from build123d import *

# Parameters (mm, degrees)
SKETCH_1_W          = 143
SKETCH_1_H          = 57.5
EXTRUDE_1_DEPTH     = 2
SKETCH_4_W          = 120
SKETCH_4_H          = 16
CUT_EXTRUDE_1_DEPTH = 10
FILLET_1_R          = 3
CUT_EXTRUDE_2_DEPTH = 10
SKETCH_6_W          = 32
SKETCH_6_H          = 16
EXTRUDE_2_DEPTH     = 2
CUT_EXTRUDE_3_DEPTH = 2
FILLET_2_R          = 3
FILLET_3_R          = 2
SKETCH_8_R          = 1.5
CUT_EXTRUDE_4_DEPTH = 78.089639382
SKETCH_10_R         = 1.721982437
CUT_EXTRUDE_5_DEPTH = 78.089639382
SKETCH_12_R         = 1.5
CUT_EXTRUDE_6_DEPTH = 78.089639382


with BuildPart() as part:
    # 草图1 → 凸台-拉伸1 (new body)
    with BuildSketch(Plane.XY):
        Rectangle(SKETCH_1_W, SKETCH_1_H)
    extrude(amount=EXTRUDE_1_DEPTH)

    # 草图4 → 切除-拉伸1 (cut)
    with BuildSketch(Plane(origin=(0, 0, 0), x_dir=(-1, 0, 0), z_dir=(0, 0, -1))):
        with Locations((0, -20.75)):
            Rectangle(SKETCH_4_W, SKETCH_4_H)
    extrude(amount=-CUT_EXTRUDE_1_DEPTH, mode=Mode.SUBTRACT)

    # 圆角1
    fillet_1_edges = [part.edges().sort_by_distance(p)[0] for p in [
        (-60, -28.75, 1),
        (60, -28.75, 1),
        (-71.5, 28.75, 1),
        (71.5, 28.75, 1),
        (71.5, -28.75, 1),
        (-71.5, -28.75, 1),
    ]]
    fillet(fillet_1_edges, radius=FILLET_1_R)

    # 草图5 → 切除-拉伸2 (cut)
    with BuildSketch(Plane.XY.offset(2)):
        with BuildLine():
            Line((4, 19.75), (4, 1.75))
            ThreePointArc((4, 1.75), (0, -2.25), (-4, 1.75))
            Line((-4, 1.75), (-4, 19.75))
            ThreePointArc((-4, 19.75), (0, 23.75), (4, 19.75))
        make_face()
        with BuildLine():
            Line((18, 19.75), (18, 1.75))
            ThreePointArc((18, 1.75), (14, -2.25), (10, 1.75))
            Line((10, 1.75), (10, 19.75))
            ThreePointArc((10, 19.75), (14, 23.75), (18, 19.75))
        make_face()
        with BuildLine():
            Line((32, 19.75), (32, 1.75))
            ThreePointArc((32, 1.75), (28, -2.25), (24, 1.75))
            Line((24, 1.75), (24, 19.75))
            ThreePointArc((24, 19.75), (28, 23.75), (32, 19.75))
        make_face()
        with BuildLine():
            Line((46, 19.75), (46, 1.75))
            ThreePointArc((46, 1.75), (42, -2.25), (38, 1.75))
            Line((38, 1.75), (38, 19.75))
            ThreePointArc((38, 19.75), (42, 23.75), (46, 19.75))
        make_face()
        with BuildLine():
            Line((60, 19.75), (60, 1.75))
            ThreePointArc((60, 1.75), (56, -2.25), (52, 1.75))
            Line((52, 1.75), (52, 19.75))
            ThreePointArc((52, 19.75), (56, 23.75), (60, 19.75))
        make_face()
        with BuildLine():
            Line((-60, 19.75), (-60, 1.75))
            ThreePointArc((-60, 1.75), (-56, -2.25), (-52, 1.75))
            Line((-52, 1.75), (-52, 19.75))
            ThreePointArc((-52, 19.75), (-56, 23.75), (-60, 19.75))
        make_face()
        with BuildLine():
            Line((-46, 19.75), (-46, 1.75))
            ThreePointArc((-46, 1.75), (-42, -2.25), (-38, 1.75))
            Line((-38, 1.75), (-38, 19.75))
            ThreePointArc((-38, 19.75), (-42, 23.75), (-46, 19.75))
        make_face()
        with BuildLine():
            Line((-32, 19.75), (-32, 1.75))
            ThreePointArc((-32, 1.75), (-28, -2.25), (-24, 1.75))
            Line((-24, 1.75), (-24, 19.75))
            ThreePointArc((-24, 19.75), (-28, 23.75), (-32, 19.75))
        make_face()
        with BuildLine():
            Line((-18, 19.75), (-18, 1.75))
            ThreePointArc((-18, 1.75), (-14, -2.25), (-10, 1.75))
            Line((-10, 1.75), (-10, 19.75))
            ThreePointArc((-10, 19.75), (-14, 23.75), (-18, 19.75))
        make_face()
    extrude(amount=-CUT_EXTRUDE_2_DEPTH, mode=Mode.SUBTRACT)

    # 草图6 → 凸台-拉伸2 (add)
    with BuildSketch(Plane(origin=(0, 0, 0), x_dir=(-1, 0, 0), z_dir=(0, 0, -1))):
        with Locations((0, -20.75)):
            Rectangle(SKETCH_6_W, SKETCH_6_H)
    extrude(amount=-EXTRUDE_2_DEPTH)

    # 草图7 → 切除-拉伸3 (cut)
    with BuildSketch(Plane(origin=(0, 0, 0), x_dir=(-1, 0, 0), z_dir=(0, 0, -1))):
        with BuildLine():
            Line((-10, -28.75), (10, -28.75))
            ThreePointArc((10, -28.75), (0, -18.75), (-10, -28.75))
        make_face()
    extrude(amount=-CUT_EXTRUDE_3_DEPTH, mode=Mode.SUBTRACT)

    # 圆角2
    fillet_2_edges = [part.edges().sort_by_distance(p)[0] for p in [
        (-60, -12.75, 1),
        (60, -12.75, 1),
        (-16, -12.75, 1),
        (-16, -28.75, 1),
        (16, -28.75, 1),
        (16, -12.75, 1),
    ]]
    fillet(fillet_2_edges, radius=FILLET_2_R)

    # 圆角3
    fillet_3_edges = [part.edges().sort_by_distance(p)[0] for p in [
        (10, -28.75, 1),
        (-10, -28.75, 1),
    ]]
    fillet(fillet_3_edges, radius=FILLET_3_R)

    # 草图8 → 切除-拉伸4 (cut, through all)
    with BuildSketch(Plane(origin=(0, 0, 0), x_dir=(-1, 0, 0), z_dir=(0, 0, -1))):
        with Locations((-68.5, 1.25)):
            Circle(SKETCH_8_R)
        with Locations((-68.5, 21.25)):
            Circle(SKETCH_8_R)
    extrude(amount=-CUT_EXTRUDE_4_DEPTH, mode=Mode.SUBTRACT)

    # 草图10 → 切除-拉伸5 (cut, through all)
    with BuildSketch(Plane(origin=(0, 0, 0), x_dir=(-1, 0, 0), z_dir=(0, 0, -1))):
        with Locations((68.5, 21.25)):
            Circle(SKETCH_10_R)
    extrude(amount=-CUT_EXTRUDE_5_DEPTH, mode=Mode.SUBTRACT)

    # 草图12 → 切除-拉伸6 (cut, through all)
    with BuildSketch(Plane(origin=(0, 0, 0), x_dir=(-1, 0, 0), z_dir=(0, 0, -1))):
        with Locations((68.5, 1.25)):
            Circle(SKETCH_12_R)
    extrude(amount=-CUT_EXTRUDE_6_DEPTH, mode=Mode.SUBTRACT)


solid = part.part
The listing builds one solid part. Answer for the finished solid, in the listing's coordinates (mm). A direction names the side the tool comes from. Round coordinates to 2 decimals unless told otherwise and drop trailing zeros. Write each loop counter-clockwise with the first axis right and the second up, starting at its lowest first coordinate (ties: lowest second). Pieces come first, ordered by that corner, then holes. Notation, with made-up numbers: M 34,31 L 71,31 A24 cw 71,48 Z; hole C 60,54 d6. An arc over 180 degrees is marked long. Write each question's results on one line, items separated by ' | '. Start each with the question number.
Item 1: The mould has two halves that part along Y. Classify faces 4 (the cylindrical face through (-66.78, 21.33, 0.99)), 5 (the cylindrical face through (41.91, 23.75, 1.01)), 6 (the cylindrical face through (-70.64, 27.85, 1.01)), 7 (the cylindrical face through (70.64, -27.85, 1.01)): +Y half, -Y half, draft (parallel to the pull), parting line (faces both ways), or undercut.
Item 2: Given pin 1 Ø1 at (x, z) = (-44.5, 1) entering from -Y; pin 2 Ø4 at (x, y) = (-68.5, 1.25) entering from -Z, each flat-ended and moving along its own axis, determine where each tip first touches the part or whether it passes through.
Item 3: Find section B-B on y = -20.5. Write down the section's boundary in (x, z).
Item 4: Find section A-A on x = 42. Write down the section's boundary in (y, z), and give its area (3 significant figures).
Item 5: Straight lines are drawn through the part: probe 1 along Y at (x, z) = (68.5, 1.3); probe 2 along Y at (x, z) = (-68.5, 1.3); probe 3 along Y at (x, z) = (-47, 1.15). For each, find the intervals that lie inside material, in ascending order.
Item 6: Which of the six approach directions +Z, -Z, +X, -X, +Y, -Y give full straight-line access (tool end or side, diameter ignored) to faces 1 (the cylindrical face through (16.9, -13.61, 1.01)), 2 (the cylindrical face through (56.09, -2.25, 1.01)), 3 (the flat face through (-1, -6, 2))?
Item 7: Find section C-C on y = 15. Give the number of separate pieces and of enclosed holes in the cut face, and give its area (3 significant figures).
Answer block:
1) face 4: undercut | face 5: undercut | face 6: +Y half | face 7: -Y half
2) pin 1: stops at y = -12.75 | pin 2: stops at z = 0
3) outline: M -71.5,0 L -60,0 L -60,2 L -71.5,2 Z; M -16,0 L -5.65,0 L -5.65,2 L -16,2 Z; M 5.65,0 L 16,0 L 16,2 L 5.65,2 Z; M 60,0 L 71.5,0 L 71.5,2 L 60,2 Z
4) outline: M -12.75,0 L -2.25,0 L -2.25,2 L -12.75,2 Z; M 23.75,0 L 28.75,0 L 28.75,2 L 23.75,2 Z | area: 31.0 mm²
5) probe 1: y = -28.75 to -0.25, 2.75 to 19.75, 22.75 to 28.75 | probe 2: y = -28.75 to -0.25, 2.75 to 19.53, 22.97 to 28.75 | probe 3: y = -12.75 to 28.75
6) face 1: +Z, -Z, -Y | face 2: +Z, -Z | face 3: +Z, +X, -X, +Y, -Y
7) separate pieces: 10 | enclosed holes: 0 | area: 142 mm²
